Geometry: final body of the model. Coordinates: model frame, mm. Round coordinates to 2 decimals unless told otherwise and drop trailing zeros. Order: outer loops, then holes, each group sorted by start corner. A loop starts at its lowest first (then second) coordinate and runs counter-clockwise, first axis right, second up. Notation, with made-up numbers: (28, 51) - (77, 51) arc R15 cw to (77, 67) - close; hole circle Ø5 at (46.25, 22). An arc over 180 degrees is marked (long way). Put each result on its own line as item: value. Start each with the question number.
(1) Section A-A (z = 10). Output: boundary loops of the cut face in (x, y).
(2) Section B-B (y = 86.5). Output: boundary loops of the cut face in (x, z), and give its area (3 significant figures).
(3) Pin query (flat end, axial travel): P1, Ø1, axis at y = 79.5, z = -7, coming from the -X side; P2, Ø2.5, axis at x = 3.54, z = 3.54, coming from the -Y side; P3, Ø3.5, axis at x = 3.54, z = 3.54, coming from the +Y side. Return the tip coordinate at first contact, or that it passes through.
(4) Material intervals for L1, parallel to Z at x = -3.25, y = 180.5; L2, parallel to Z at x = -1.75, y = 251.5; L3, parallel to X at y = 188, z = 4.5, sorted ascending. Write a range as [from, to].
Autodesk Inventor part; units mm, degrees
ref_plane "YZ Plane" through (0, 0, 0) normal (1, 0, 0) x (0, 1, 0)
ref_plane "XZ Plane" through (0, 0, 0) normal (0, 1, 0) x (-1, 0, 0)
ref_plane "XY Plane" through (0, 0, 0) normal (0, 0, 1) x (1, 0, 0)
sketch "Sketch1" plane through (0, 0, 0) normal (0, 1, 0) x (-1, 0, 0)
  circle A0 centre (0, 0) radius 12.5
  dimension "d0" = 25
extrude "Extrusion1" add sketch "Sketch1" along normal blind 280
sketch "Sketch2" plane through (0, 0, 0) normal (0, -1, 0) x (1, 0, 0)
  line L0 (-3.5355, -3.5355) -> (3.5355, 3.5355)
  line L1 (-3.5355, -3.5355) -> (6.4645, -3.5355) construction
  circle A0 centre (-3.5355, -3.5355) radius 1.9
  circle A1 centre (3.5355, 3.5355) radius 1.9
  point P0 (0, 0)
  dimension "d3" = 10
  dimension "d4" = 45
  dimension "d5" = 3.8
  dimension "d6" = 3.8
extrude "Extrusion2" cut sketch "Sketch2" against normal blind 40
sketch "Sketch3" plane through (0, 0, 0) normal (0, -1, 0) x (1, 0, 0)
  line L0 (0, 0) -> (-4.2426, 4.2426)
  line L1 (0, 0) -> (6, 0) construction
  circle A0 centre (-4.2426, 4.2426) radius 3
  dimension "d9" = 6
  dimension "d10" = 135
  dimension "d11" = 6
extrude "Extrusion3" cut sketch "Sketch3" against normal through all
sketch "Sketch6" plane through (0, 280, 0) normal (0, 1, 0) x (1, 0, 0)
  circle A0 centre (-3.5355, -3.5355) radius 1.9 construction
  circle A1 centre (3.5355, 3.5355) radius 1.9 construction
  line L0 (-3.5355, 3.5355) -> (3.5355, -3.5355)
  line L1 (-3.5355, 3.5355) -> (6.4645, 3.5355) construction
  circle A2 centre (3.5355, -3.5355) radius 2
  circle A3 centre (-3.5355, 3.5355) radius 2
  point P0 (0, 0)
  dimension "d16" = 10
  dimension "d17" = 45
  dimension "d18" = 4
  dimension "d19" = 4
extrude "Extrusion4" cut sketch "Sketch6" against normal blind 8
properties part number "Dowel2"
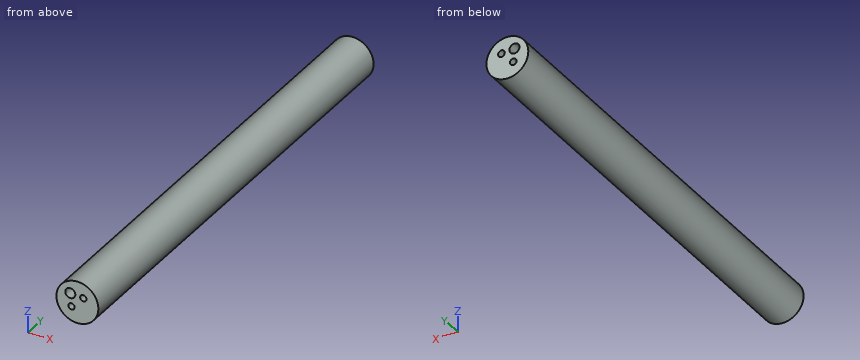
Checks:
1. outline: (-7.5, 0) - (7.5, 0) - (7.5, 280) - (-7.5, 280) - close
2. outline: circle Ø25 at (0, 0); hole circle Ø6 at (-4.24, 4.24)
2. area: 463 mm²
3. P1: stops at x = -10.68
3. P2: stops at y = 40
3. P3: stops at y = 272
4. L1: z = [-12.07, 1.41], [7.07, 12.07]
4. L2: z = [-12.38, 2.57], [5.91, 12.38]
4. L3: x = [-11.66, -7.23], [-1.25, 11.66]
